Input: part model. Units: mm. Frame: model coordinates. A direction names the side the tool comes from. Give positions to 0.01 mm unless a question says otherwise; leave off trailing zeros. Loops run counter-clockwise (first coordinate to the right, second up) from the corner with the lowest first, then second, coordinate; pieces in that order, holes last. Notation, with made-up numbers: (88, 3) -> (114, 3) arc R30 ccw to (114, 27) -> close; hole circle Ø9 at (60, -6). An arc over 180 degrees is marked (long way). Answer as a JSON object with one key per item and string values.
```python
from build123d import *

# Parameters (mm, degrees)
F1_DEPTH = 12
F2_T     = -1
F4_W     = 12
F4_H     = 11
F4_W_2   = 8.5
F5_DEPTH = 5


with BuildPart() as f1:
    # F0 (on Top) → F1 (new body)
    with BuildSketch(Plane.XY):
        Polygon((28.25, 34), (-28.25, 34), (-28.25, -34), (-25.25, -34), (15.75, -34), (28.25, -34), align=None)
        Polygon((15.75, -34), (-25.25, -34), (-21.0784263909, -37), (11.9215736091, -37), align=None)
    extrude(amount=F1_DEPTH)

    # F2
    f2_openings = [f1.faces().sort_by_distance(p)[0] for p in [
        (-0.131058, -0.99532, 12),
    ]]
    offset(amount=F2_T, openings=f2_openings, kind=Kind.INTERSECTION)

    # F4 (on offset) → F5 (cut)
    with BuildSketch(Plane.XZ.offset(-34)):
        with Locations((10.75, 9.8824445456)):
            Rectangle(F4_W, F4_H)
        with Locations((-19.5, 10.0444257557)):
            Rectangle(F4_W_2, F4_H)
    extrude(amount=F5_DEPTH, mode=Mode.SUBTRACT)


solid = f1.part
```
Q1. Section A-A, the plane z = 9.5. Return the cut outline in (x, y), then the cut area to 3 significant figures.
Evaluation:
{"outline": "(-28.25, -34) -> (-25.25, -34) -> (-21.08, -37) -> (11.92, -37) -> (15.75, -34) -> (28.25, -34) -> (28.25, 34) -> (16.75, 34) -> (16.75, 33) -> (27.25, 33) -> (27.25, -33) -> (15.4, -33) -> (11.58, -36) -> (-20.76, -36) -> (-24.93, -33) -> (-27.25, -33) -> (-27.25, 33) -> (-23.75, 33) -> (-23.75, 34) -> (-28.25, 34) -> close; (-15.25, 33) -> (4.75, 33) -> (4.75, 34) -> (-15.25, 34) -> close", "area": "227 mm2"}
Q2. Ray query, line 1 along X through (y, z) = (-24.5, 8.5); line 2 along Y through (x, z) = (3.5, 7.25); line 3 along Y through (x, z) = (23, 4.25). Return the intervals inside material, ascending.
Evaluation:
{"line 1": "x = -28.25 to -27.25, 27.25 to 28.25", "line 2": "y = -37 to -36, 33 to 34", "line 3": "y = -34 to -33, 33 to 34"}
Q3. Draft query along X for faces 1 (the flat face through (-27, -34, 6)), 2 (the flat face through (-23.19, -35.48, 5.92)), 3 (the flat face through (-27.25, 0, 6)). Return one class per face: +X half, -X half, draft (parallel to the pull), parting line (faces both ways), or undercut.
Evaluation:
{"face 1": "draft", "face 2": "-X half", "face 3": "undercut"}
Q4. Access query for faces 4 (the flat face through (22, -34, 6)), 5 (the flat face through (0, -1, 0)), 6 (the flat face through (13.464, -34.521, 6.423)). Directions: +Z, -Z, +X, -X, +Y, -Y. A direction counts if a zero-diameter tool reaches every point of the face in a straight line with its end or side. Return the directions, or none.
Evaluation:
{"face 4": "+Z, -Z, +X, -Y", "face 5": "-Z, +X, -X, +Y, -Y", "face 6": "+Z"}
Q5. Section B-B, the plane x = -17. Return the cut outline in (y, z), then the cut area to 3 significant figures.
Evaluation:
{"outline": "(-37, 0) -> (34, 0) -> (34, 4.54) -> (33, 4.54) -> (33, 1) -> (-36, 1) -> (-36, 12) -> (-37, 12) -> close", "area": "85.5 mm2"}
Q6. Section D-D, the plane z = 3.25. Return the cut outline in (x, y), then the cut area to 3 significant figures.
Evaluation:
{"outline": "(-28.25, -34) -> (-25.25, -34) -> (-21.08, -37) -> (11.92, -37) -> (15.75, -34) -> (28.25, -34) -> (28.25, 34) -> (-28.25, 34) -> close; hole (-27.25, -33) -> (-24.93, -33) -> (-20.76, -36) -> (11.58, -36) -> (15.4, -33) -> (27.25, -33) -> (27.25, 33) -> (-27.25, 33) -> close", "area": "247 mm2"}
Q7. Pin query (flat end, axial travel): pin 1 (2 mm diameter, centred on x = -22.5, y = -7, fed in from +Z); pin 2 (0.9 mm diameter, centred on x = -27, z = 4.5, fed in from -Y); pin 3 (1.1 mm diameter, centred on x = -19.5, y = 33.5, fed in from +Z). Return the tip coordinate at first contact, or that it passes through.
Evaluation:
{"pin 1": "stops at z = 1", "pin 2": "stops at y = -34", "pin 3": "stops at z = 4.54"}
Q8. Section C-C, the plane y = 14.5. Return the cut outline in (x, z).
Evaluation:
{"outline": "(-28.25, 0) -> (28.25, 0) -> (28.25, 12) -> (27.25, 12) -> (27.25, 1) -> (-27.25, 1) -> (-27.25, 12) -> (-28.25, 12) -> close"}
